```python
from build123d import *

# Parameters (mm, degrees)
SKETCH_1_W                  = 52
SKETCH_1_H                  = 23
EXTRUDE_1_DEPTH             = 16
HOLE_WIZARD_6_6_6_6_1_D     = 6.6
HOLE_WIZARD_6_6_6_6_1_DEPTH = 16


with BuildPart() as part:
    # 草图1 → 凸台-拉伸1 (new body)
    with BuildSketch(Plane.XY):
        Rectangle(SKETCH_1_W, SKETCH_1_H)
    extrude(amount=EXTRUDE_1_DEPTH)

    # Ø6.6 (6.6) 直径孔1
    with Locations(Plane.XY.offset(16)):
        with Locations((-19, 0), (19, 0)):
            Hole(HOLE_WIZARD_6_6_6_6_1_D / 2, depth=HOLE_WIZARD_6_6_6_6_1_DEPTH)


solid = part.part
```
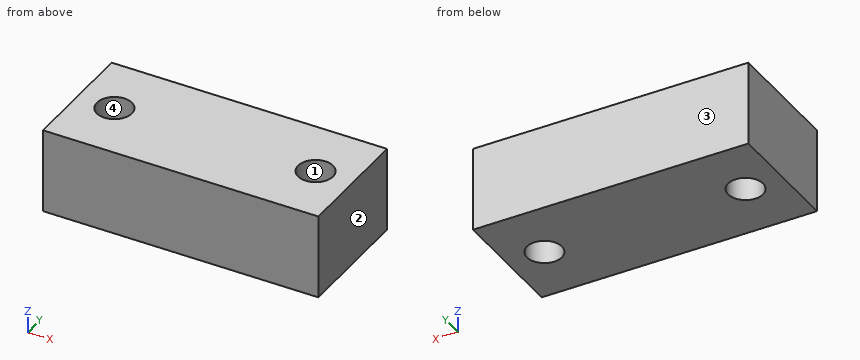
The model under review builds one solid part; all positions refer to its coordinate system, in mm. Face numbers are marked on the shaded views. Round coordinates to 2 decimals unless told otherwise and drop trailing zeros. Write each loop counter-clockwise with the first axis right and the second up, starting at its lowest first coordinate (ties: lowest second). Pieces come first, ordered by that corner, then holes. Notation, with made-up numbers: (23, 4.25) - (53, 4.25) arc R21 ccw to (53, 39.25) - close; hole circle Ø10 at (86, 32). An arc over 180 degrees is marked (long way). Answer as CSV lines item,"result". Start each with the question number.
(1) We need section A-A on y = 0. State the section outline as (x, z) points, plus the area to 3 significant figures.
(2) We need section B-B on x = -19. State the section outline as (y, z) points.
(3) We need section C-C on z = 14.75. State the section outline as (x, y) points.
(4) To check wall thickness, follow line 1 (X direction, y = 0.25, z = 8); line 2 (Y direction, x = -19, z = 10.75); line 3 (Y direction, x = -18, z = 0.5). State the ranges of each line that lie inside material, in increasing order.
(5) Draft analysis for pull direction X (two halves, no side actions). For the marked faces 1, 2, 3 and 4, state which applies: pulls with the +X half, pulls with the -X half, needs draft (parallel to the pull), parting line crosses it, or undercut.
(6) For pin 1 Ø5.5 at (x, y) = (19, 0) entering from +Z, flat-tipped, find the tip position at first contact; note if it passes through.
(7) We need section D-D on x = 17. State the section outline as (y, z) points, plus the area to 3 significant figures.
Worked answers:
1,outline,"(-26, 0) - (-22.3, 0) - (-22.3, 16) - (-26, 16) - close; (-15.7, 0) - (15.7, 0) - (15.7, 16) - (-15.7, 16) - close; (22.3, 0) - (26, 0) - (26, 16) - (22.3, 16) - close"
1,area,"621 mm²"
2,outline,"(-11.5, 0) - (-3.3, 0) - (-3.3, 16) - (-11.5, 16) - close; (3.3, 0) - (11.5, 0) - (11.5, 16) - (3.3, 16) - close"
3,outline,"(-26, -11.5) - (26, -11.5) - (26, 11.5) - (-26, 11.5) - close; hole circle Ø6.6 at (-19, 0); hole circle Ø6.6 at (19, 0)"
4,line 1,"-26 to -22.29, -15.71 to 15.71, 22.29 to 26"
4,line 2,"-11.5 to -3.3, 3.3 to 11.5"
4,line 3,"-11.5 to -3.14, 3.14 to 11.5"
5,face 1,"undercut"
5,face 2,"pulls with the +X half"
5,face 3,"needs draft"
5,face 4,"undercut"
6,pin 1,"through"
7,outline,"(-11.5, 0) - (-2.62, 0) - (-2.62, 16) - (-11.5, 16) - close; (2.62, 0) - (11.5, 0) - (11.5, 16) - (2.62, 16) - close"
7,area,"284 mm²"
